Check sheet for the modelled part. Datum: model origin and axes. Units: mm. Face numbers are marked on the shaded views. A direction names the side the tool comes from. Coordinates: 2 decimals unless noted, no trailing zeros. Loops run counter-clockwise (first coordinate to the right, second up) from the corner with the lowest first, then second, coordinate; pieces in that order, holes last. Notation, with made-up numbers: (-13.5, 49) - (24.5, 49) arc R13 cw to (24.5, 58) - close; hole circle Ø5 at (-23, 29.5). An arc over 180 degrees is marked (long way). Write each question's results on one line, items separated by ' | '. Start each with the question number.
1. Cross-section at B-B (y = 26.25). Record the cut outline in (x, z).
2. Tool access check on the marked faces 1 and 2. Record the directions out of +Z, -Z, +X, -X, +Y, -Y that give a thin tool (end or side, any length) a straight path to the whole face; none if there is none.
3. Thickness scan on line 1 (Y direction, x = -36.5, z = 0); line 2 (X direction, y = 22, z = -15); line 3 (Y direction, x = -22, z = 9). Record the ranges inside material, lowest first. Write a range as [from, to].
4. Gauge pin test, flat end, axial feed: P1, Ø3, axis at x = 1, z = 15, coming from the +Y side. Record the tip position at first contact, or that the pin passes through.
5. Cross-section at D-D (y = 20.5). Record the cut outline in (x, z).
6. Draft check along X on the marked faces 3, 4, 5 and 6. Enter one of: released by +X, released by -X, zero draft, split by the parting line, or undercut.
7. Cross-section at C-C (z = 9). Record the cut outline in (x, y), and give its area (3 significant figures).
8. Cross-section at A-A (z = 0.5). Record the cut outline in (x, y), and give its area (3 significant figures).
```python
from build123d import *

# Parameters (mm, degrees)
SKETCH2_W           = 80
SKETCH2_H           = 50
BOSS_EXTRUDE1_DEPTH = 8
SKETCH3_R           = 1.3
BOSS_EXTRUDE2_DEPTH = 8


with BuildPart() as part:
    # Sketch2 → Boss-Extrude1 (new body)
    with BuildSketch(Plane(origin=(0, 0, 0), x_dir=(1, 0, 0), z_dir=(0, 1, 0))):
        Rectangle(SKETCH2_W, SKETCH2_H)
    extrude(amount=BOSS_EXTRUDE1_DEPTH)

    # Sketch3 → Boss-Extrude2 (add)
    with BuildSketch(Plane(origin=(40, 0, 0), x_dir=(0, 0, -1), z_dir=(1, 0, 0))):
        Polygon((13.758286246, 28), (25, 8), (-25, 8), (-13.758286246, 28), align=None)
        with Locations((0, 23)):
            Circle(SKETCH3_R, mode=Mode.SUBTRACT)
    boss_extrude2 = extrude(amount=-BOSS_EXTRUDE2_DEPTH)

    # Mirror1: Boss-Extrude2 across plane
    add(boss_extrude2.mirror(Plane(origin=(0, 0, 0), x_dir=(0, 0, 1), z_dir=(1, 0, 0))))


solid = part.part
```
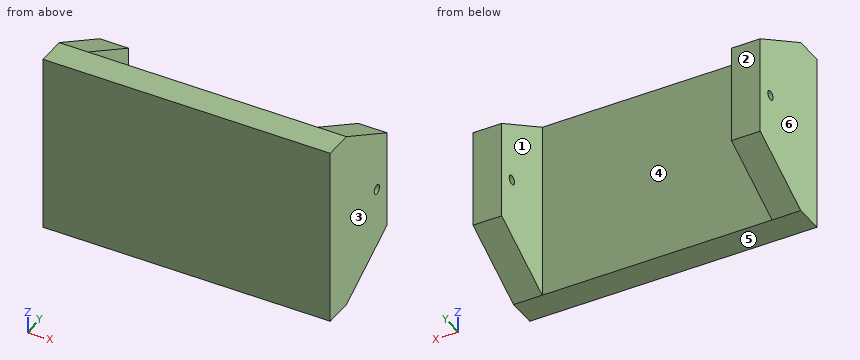
Established:
1) outline: (-40, -14.74) - (-32, -14.74) - (-32, 14.74) - (-40, 14.74) - close; (32, -14.74) - (40, -14.74) - (40, 14.74) - (32, 14.74) - close
2) face 1: +Z, -Z, +Y | face 2: +Z, -Z, +X, -X, +Y
3) line 1: [0, 21.7], [24.3, 28] | line 2: [-40, -32], [32, 40] | line 3: [0, 8]
4) P1: y = 8
5) outline: (-40, -17.97) - (-32, -17.97) - (-32, 17.97) - (-40, 17.97) - close; (32, -17.97) - (40, -17.97) - (40, 17.97) - (32, 17.97) - close
6) face 3: released by +X | face 4: undercut | face 5: zero draft | face 6: released by -X
7) outline: (-40, 0) - (40, 0) - (40, 28) - (32, 28) - (32, 8) - (-32, 8) - (-32, 28) - (-40, 28) - close | area: 960 mm^2
8) outline: (-40, 0) - (40, 0) - (40, 21.8) - (32, 21.8) - (32, 8) - (-32, 8) - (-32, 21.8) - (-40, 21.8) - close; (-40, 24.2) - (-32, 24.2) - (-32, 28) - (-40, 28) - close; (32, 24.2) - (40, 24.2) - (40, 28) - (32, 28) - close | area: 922 mm^2
